from build123d import *

# Parameters (mm, degrees)
F1_DEPTH = 100.076
F3_DEPTH = 48.26


with BuildPart() as f1:
    # F0 (on Front) → F1 (new body)
    with BuildSketch(Plane.XZ):
        Polygon((0, 22.108026), (0, 0), (66.624872, 0), align=None)
    extrude(amount=F1_DEPTH)

    # F2 (on face) → F3 (cut)
    with BuildSketch(Plane(origin=(6.608418, 0, 19.915165), x_dir=(0.949111, 0, -0.314942), z_dir=(0.314942, 0, 0.949111))):
        with BuildLine():
            ThreePointArc((28.135825, -7.469715), (15.726606, -12.609782), (10.58654, -25.019))
            Line((10.58654, -25.019), (10.58654, -75.057))
            ThreePointArc((10.58654, -75.057), (28.135825, -92.606285), (45.685109, -75.057))
            Line((45.685109, -75.057), (45.685109, -25.019))
            ThreePointArc((45.685109, -25.019), (40.545043, -12.609782), (28.135825, -7.469715))
        make_face()
    extrude(amount=-F3_DEPTH, mode=Mode.SUBTRACT)


solid = f1.part
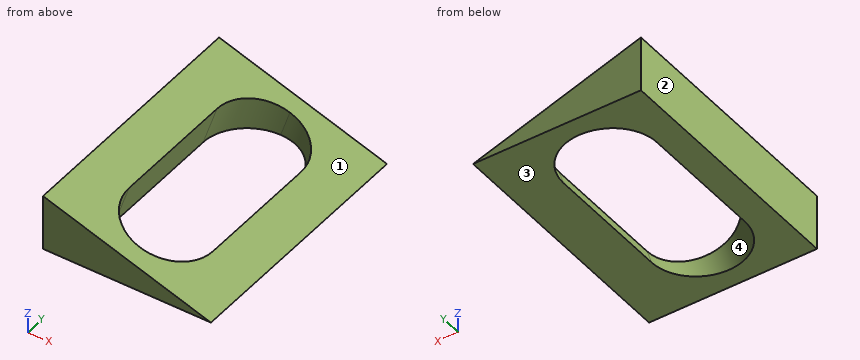
Geometry check sheet. Reference: the model listing, model coordinates, mm. Face numbers are marked on the shaded views. Coordinates: 2 decimals unless noted, no trailing zeros. Loops run counter-clockwise (first coordinate to the right, second up) from the corner with the lowest first, then second, coordinate; pieces in that order, holes last. Notation, with made-up numbers: (47, 74) - (94, 74) arc R11 ccw to (94, 84) - close; hole circle Ø7 at (40, 54). An arc over 180 degrees is marked (long way). Use one line per item in the form item = value. Start each with the question number.
Item 1: Mould release check, pull along X, two halves, no side actions. Record for the marked faces 1, 2, 3 and 4: +X half, -X half, draft (parallel to the pull), parting line (faces both ways), or undercut.
Item 2: Thickness scan on probe 1 along Y at (x, z) = (29, 4.25); probe 2 along Y at (x, z) = (28.5, 8.5); probe 3 along Z at (x, y) = (7, -81.5). Record the ranges inside material, lowest first.
Item 3: Section check A-A, the plane y = -58.5. Enter the section's corners in (x, z).
Item 4: Section check D-D, the plane x = 60. Enter the section's corners in (y, z), and give its area (3 significant figures).
Item 5: Gauge pin test, flat ends, axial feed: pin 1 (4 mm diameter, centred on x = 55, y = -19, fed in from +Z); pin 2 (6 mm diameter, centred on x = 35.5, z = 7, fed in from +Y); pin 3 (5 mm diameter, centred on x = 48.5, z = 11, fed in from -Y); pin 4 (6 mm diameter, centred on x = 51.5, y = -63, fed in from +Z). Record the tip position at first contact, or that the pin passes through.
Item 6: Section check B-B, the plane y = -20.5. Enter the section's corners in (x, z).
Item 7: Section check C-C, the plane z = 20.75. Enter the section's corners in (x, y), and give its area (3 significant figures).
Computed:
q1.face_1 = +X half
q1.face_2 = -X half
q1.face_3 = draft
q1.face_4 = undercut
q2.probe_1 = -100.08 to -92.5, -7.58 to 0
q2.probe_2 = -100.08 to -92.2, -7.88 to 0
q2.probe_3 = 0 to 19.79
q3.outline = (0, 0) - (11.15, 0) - (16.66, 16.58) - (0, 22.11) - close; (48.13, 0) - (66.62, 0) - (49.97, 5.53) - close
q4.outline = (-100.08, 0) - (0, 0) - (0, 2.2) - (-100.08, 2.2) - close
q4.area = 220 mm2
q5.pin_1 = 4.52
q5.pin_2 = 0
q5.pin_3 = through
q5.pin_4 = 5.53
q6.outline = (0, 0) - (11.78, 0) - (17.22, 16.39) - (0, 22.11) - close; (47.51, 0) - (66.62, 0) - (49.41, 5.71) - close
q7.outline = (0, -100.08) - (4.09, -100.08) - (4.09, 0) - (0, 0) - close
q7.area = 410 mm2
